from build123d import *

# Parameters (mm, degrees)
EXTRUDE_410_DEPTH         = 2.5
HOLE_WIZARD_M6_AT_2_COUNT = 2
HOLE_WIZARD_M6_AT_2_PITCH = 130
FILLET_1_R                = 10
SKETCH_2_R                = 5
CUT_EXTRUDE_1_DEPTH       = 212.621774622


with BuildPart() as part:
    # Эскиз1 → Extrude 410 (new, symmetric)
    with BuildSketch(Plane.XY):
        Polygon((0, 0), (160, 0), (40, 150), (0, 150), align=None)
    extrude(amount=EXTRUDE_410_DEPTH, both=True)

    # Эскиз4 → Крепление-M6 (revolve, cut)
    with BuildSketch(Plane(origin=(14, 140, 2.5), x_dir=(0, -1, 0), z_dir=(1, 0, 0))):
        Polygon((0, 0), (0, 5), (3.3, 5), (3.3, 3), (6.3, 0), align=None)
    hole_wizard_m6 = revolve(axis=Axis((14, 140, 8.85), (0, 0, -1)), mode=Mode.SUBTRACT)

    # Крепление-M6 at 2: Крепление-M6 ×2
    with Locations(*[(0, -i * HOLE_WIZARD_M6_AT_2_PITCH, 0) for i in range(1, HOLE_WIZARD_M6_AT_2_COUNT)]):
        add(hole_wizard_m6, mode=Mode.SUBTRACT)

    # Скругление1
    fillet_1_edges = [part.edges().sort_by_distance(p)[0] for p in [
        (0, 150, 0),
        (40, 150, 0),
        (160, 0, 0),
        (0, 0, 0),
    ]]
    fillet(fillet_1_edges, radius=FILLET_1_R)

    # Эскиз2 → Вырез-Вытянуть1 (cut, through all)
    with BuildSketch(Plane.XY.offset(2.5)):
        with Locations((139.193751525, 10)):
            Circle(SKETCH_2_R)
        with Locations((29.193751525, 10)):
            Circle(SKETCH_2_R)
    extrude(amount=-CUT_EXTRUDE_1_DEPTH, mode=Mode.SUBTRACT)


solid = part.part
Geometry: final body of the model. Coordinates: model frame, mm. Coordinates: 2 decimals unless noted, no trailing zeros. Order: outer loops, then holes, each group sorted by start corner. A loop starts at its lowest first (then second) coordinate and runs counter-clockwise, first axis right, second up.
1) Section C-C (y = 125). Return loops of the section in (x, z).
Result sheet:
outline: (0, -2.5) - (60, -2.5) - (60, 2.5) - (0, 2.5) - close
2) Section A-A (z = 1.05). Return loops of the section in (x, y).
Result sheet:
outline: (0, 10) arc R10 ccw to (10, 0) - (139.19, 0) arc R10 ccw to (147, 16.25) - (43, 146.25) arc R10 ccw to (35.19, 150) - (10, 150) arc R10 ccw to (0, 140) - close; hole circle Ø9.7 at (14, 10); hole circle Ø9.7 at (14, 140); hole circle Ø10 at (29.19, 10); hole circle Ø10 at (139.19, 10)
3) Section D-D (x = 117). Return loops of the section in (y, z), then the cut area to 3 significant figures.
Result sheet:
outline: (0, -2.5) - (53.75, -2.5) - (53.75, 2.5) - (0, 2.5) - close
area: 269 mm2
4) Section B-B (x = 14). Return loops of the section in (y, z), then the cut area to 3 significant figures.
Result sheet:
outline: (0, -2.5) - (6.7, -2.5) - (6.7, -0.5) - (3.7, 2.5) - (0, 2.5) - close; (13.3, -2.5) - (136.7, -2.5) - (136.7, -0.5) - (133.7, 2.5) - (16.3, 2.5) - (13.3, -0.5) - close; (143.3, -2.5) - (150, -2.5) - (150, 2.5) - (146.3, 2.5) - (143.3, -0.5) - close
area: 666 mm2
5) Draft query along X for faces 1 (the cylindrical face through (2.85, 146.99, -0.04)), 2 (the flat face through (96, 80, 0)), 3 (the cylindrical face through (13.9, 13.3, -1.5)). Return one class per face: released by +X, released by -X, zero draft, split by the parting line, or undercut.
Result sheet:
face 1: released by -X
face 2: released by +X
face 3: undercut
6) First-contact query: P1, Ø8.5, axis at x = 14, y = 10, coming from the +Z side; P2, Ø2, axis at y = 130, z = -1.5, coming from the +X side; P3, Ø6, axis at x = 29.19, y = 10, coming from the -Z side; P4, Ø10.5, axis at x = 14, y = 140, coming from the -Z side. Flat tips, straight axial feed; report the tip coordinate or a pass-through.
Result sheet:
P1: stops at z = 0.45
P2: stops at x = 56.8
P3: passes through
P4: stops at z = -2.5
7) Ray query, probe 1 along Y at (x, z) = (14, -1.8); probe 2 along X at (y, z) = (140, -1.5); probe 3 along Y at (x, z) = (33.5, -0.7). Return the intervals inside material, ascending.
Result sheet:
probe 1: y = 0 to 6.7, 13.3 to 136.7, 143.3 to 150
probe 2: x = 0 to 10.7, 17.3 to 48
probe 3: y = 0 to 7.46, 12.54 to 150
